from build123d import *
from OCP.BRepFilletAPI import BRepFilletAPI_MakeChamfer

# Parameters (mm, degrees)
SKICA1_W                = 100
SKICA1_H                = 80
SKICA1_W_2              = 46.8
SKICA1_H_2              = 36.8
SKICA1_H_3              = 76.8
P_IDAT_VYSUNUT_M1_DEPTH = 20
SKICA1_6_W              = 104
SKICA1_6_H              = 84
P_IDAT_VYSUNUT_M3_DEPTH = 1.6
SKICA1_7_W              = 104
SKICA1_7_H              = 84
SKICA1_7_W_2            = 100
SKICA1_7_H_2            = 80
P_IDAT_VYSUNUT_M4_DEPTH = 6
ZKOSEN_14_SIZE          = 2
ZKOSEN_14_SIZE_2        = 5


with BuildPart() as part:
    # Skica1 → Přidat vysunutím1 (new body)
    with BuildSketch(Plane(origin=(0, 0, 0), x_dir=(1, 0, 0), z_dir=(0, 1, 0))):
        Rectangle(SKICA1_W, SKICA1_H)
        with Locations((-25, 20)):
            Rectangle(SKICA1_W_2, SKICA1_H_2, mode=Mode.SUBTRACT)
        with Locations((-25, -20)):
            Rectangle(SKICA1_W_2, SKICA1_H_2, mode=Mode.SUBTRACT)
        with Locations((25, 0)):
            Rectangle(SKICA1_W_2, SKICA1_H_3, mode=Mode.SUBTRACT)
    extrude(amount=P_IDAT_VYSUNUT_M1_DEPTH)

    # Skica1<6> → Přidat vysunutím3 (add)
    with BuildSketch(Plane(origin=(0, 0, 0), x_dir=(1, 0, 0), z_dir=(0, 1, 0))):
        Rectangle(SKICA1_6_W, SKICA1_6_H)
    extrude(amount=P_IDAT_VYSUNUT_M3_DEPTH)

    # Skica1<7> → Přidat vysunutím4 (add)
    with BuildSketch(Plane(origin=(0, 0, 0), x_dir=(1, 0, 0), z_dir=(0, 1, 0))):
        Rectangle(SKICA1_7_W, SKICA1_7_H)
        Rectangle(SKICA1_7_W_2, SKICA1_7_H_2, mode=Mode.SUBTRACT)
    extrude(amount=P_IDAT_VYSUNUT_M4_DEPTH)

    # Zkosení14
    zkosen_14_edges_1 = [part.edges().sort_by_distance(p)[0] for p in [
        (52, 6, 0),
    ]]
    zkosen_14_side_1 = [part.faces().sort_by_distance(p)[0] for p in [
        (51.96, 6, 0),
    ]]
    zkosen_14_edges_2 = [part.edges().sort_by_distance(p)[0] for p in [
        (0, 6, -42),
    ]]
    zkosen_14_side_2 = [part.faces().sort_by_distance(p)[0] for p in [
        (0, 6, -41.96),
    ]]
    zkosen_14_edges_3 = [part.edges().sort_by_distance(p)[0] for p in [
        (-52, 6, 0),
    ]]
    zkosen_14_side_3 = [part.faces().sort_by_distance(p)[0] for p in [
        (-52, 5.96, 0),
    ]]
    zkosen_14_edges_4 = [part.edges().sort_by_distance(p)[0] for p in [
        (0, 6, 42),
    ]]
    zkosen_14_side_4 = [part.faces().sort_by_distance(p)[0] for p in [
        (0, 6, 41.96),
    ]]
    zkosen_14 = BRepFilletAPI_MakeChamfer(part.part.solid().wrapped)
    for e in zkosen_14_edges_1:
        zkosen_14.Add(ZKOSEN_14_SIZE - 0.0001, ZKOSEN_14_SIZE_2 - 0.0001, e.wrapped, zkosen_14_side_1[0].wrapped)
    for e in zkosen_14_edges_2:
        zkosen_14.Add(ZKOSEN_14_SIZE - 0.0001, ZKOSEN_14_SIZE_2 - 0.0001, e.wrapped, zkosen_14_side_2[0].wrapped)
    for e in zkosen_14_edges_3:
        zkosen_14.Add(ZKOSEN_14_SIZE_2 - 0.0001, ZKOSEN_14_SIZE - 0.0001, e.wrapped, zkosen_14_side_3[0].wrapped)
    for e in zkosen_14_edges_4:
        zkosen_14.Add(ZKOSEN_14_SIZE - 0.0001, ZKOSEN_14_SIZE_2 - 0.0001, e.wrapped, zkosen_14_side_4[0].wrapped)
    add(Compound.cast(zkosen_14.Shape()), mode=Mode.REPLACE)  # a hair under: the kernel refuses the full size


solid = part.part
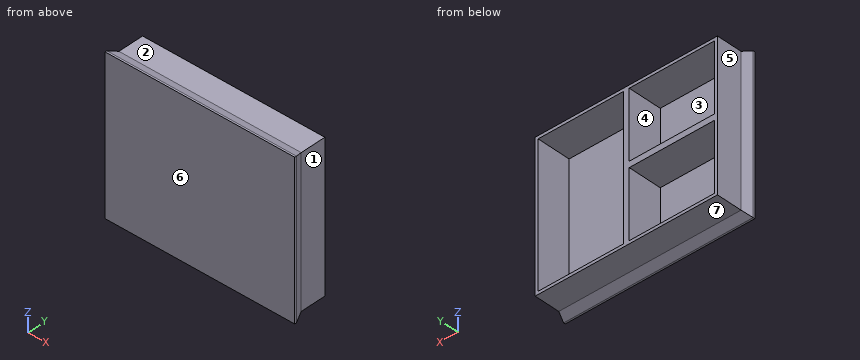
The model under review builds one solid part; all positions refer to its coordinate system, in mm. Face numbers are marked on the shaded views. A direction names the side the tool comes from. Give positions to 0.01 mm unless a question says otherwise; leave off trailing zeros. Order: outer loops, then holes, each group sorted by start corner. A loop starts at its lowest first (then second) coordinate and runs counter-clockwise, first axis right, second up. Notation, with made-up numbers: M 5,11.25 L 45,11.25 A26 cw 45,37.25 Z; hole C -36,3.25 d1. An arc over 180 degrees is marked long. Use one line per item in the form item = value. Start each with the question number.
Item 1: For the marked faces 4, 5, 6 and 7, list the 3-axis set-ups (+Z, -Z, +X, -X, +Y, -Y) from which the entire face can be reached by the end or side of a thin tool; tool diameter is ignored.
Item 2: Insertion check: pin 1 Ø11 at (x, y) = (17, 14) entering from -Z; pin 2 Ø5.5 at (x, y) = (-18.5, 11.5) entering from +Z; pin 3 Ø8 at (y, z) = (9, -3.5) entering from +X. Each pin has a flat end and moves straight along its axis. Give the tip position at first contact, or say it passes through.
Item 3: To check wall thickness, follow line 1 along Z through (x, y) = (-6, 7); line 2 along X through (y, z) = (10.25, -31.5); line 3 along Z through (x, y) = (12, 10). State the ranges of each line that lie inside material, in increasing order. Write a range as from..to.
Item 4: We need section A-A on y = 10. Give the boundary of the cut face in (x, z).
Item 5: We need section D-D on y = 3.5. Give the boundary of the cut face in (x, z).
Item 6: The part is to be moulded in two halves that separate along X. For the marked faces 1, 2 and 3, say which applies: pulls with the +X half, pulls with the -X half, needs draft (parallel to the pull), parting line crosses it, or undercut.
Completed:
q1.face_4 = +Y
q1.face_5 = +Z, -Z, -X, +Y
q1.face_6 = +Z, -Z, +X, -X, -Y
q1.face_7 = -Z, +X, -X, +Y
q2.pin_1 = -40
q2.pin_2 = 40
q2.pin_3 = 50.4
q3.line_1 = -40..-38.4, -1.6..1.6, 38.4..40
q3.line_2 = -50..-48.4, -1.6..1.6, 48.4..50
q3.line_3 = -40..-38.4, 38.4..40
q4.outline = M -50,-40 L 50,-40 L 50,40 L -50,40 Z; hole M -48.4,-38.4 L -1.6,-38.4 L -1.6,-1.6 L -48.4,-1.6 Z; hole M -48.4,1.6 L -1.6,1.6 L -1.6,38.4 L -48.4,38.4 Z; hole M 1.6,-38.4 L 48.4,-38.4 L 48.4,38.4 L 1.6,38.4 Z
q5.outline = M -51,-41 L 51,-41 L 51,41 L -51,41 Z; hole M -48.4,-38.4 L -1.6,-38.4 L -1.6,-1.6 L -48.4,-1.6 Z; hole M -48.4,1.6 L -1.6,1.6 L -1.6,38.4 L -48.4,38.4 Z; hole M 1.6,-38.4 L 48.4,-38.4 L 48.4,38.4 L 1.6,38.4 Z
q6.face_1 = pulls with the +X half
q6.face_2 = needs draft
q6.face_3 = undercut
